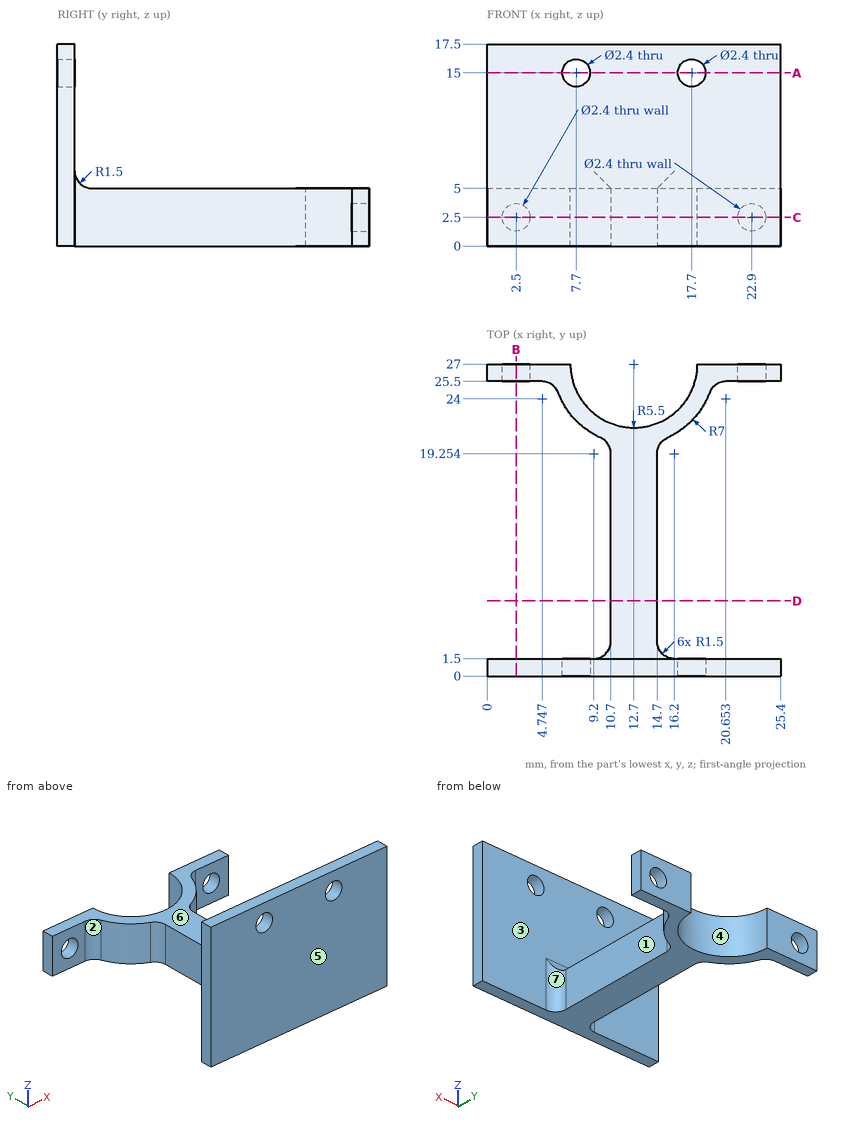
Geometry: see drawing. Coordinates: mm, zero at the bounding-box minimum. A direction names the side the tool comes from. Coordinates: 2 decimals unless noted, no trailing zeros. Order: outer loops, then holes, each group sorted by start corner. A loop starts at its lowest first (then second) coordinate and runs counter-clockwise, first axis right, second up. Notation, with made-up numbers: M 19,30.25 L 52,30.25 A10 cw 52,44.25 Z; hole C 3.5,79.5 d4. An arc over 180 degrees is marked long. Answer in a Markdown table with one row per item. Add a question column.
Q1. Section query D-D on y = 6.5. Return the cut outline in (x, z), and give its area (3 significant figures).
Q2. Section query B-B on x = 2.5. Return the cut outline in (y, z).
Q3. Contact query for flat-ended pins moving along their axis: P1, Ø5, axis at x = 4.5, z = 10, coming from the -Y side; P2, Ø1.5, axis at y = 12, z = 1.5, coming from the +X side; P3, Ø2, axis at x = 8.5, z = 11.5, coming from the +Y side; P4, Ø1.9, axis at x = 7.7, z = 15, coming from the +Y side. Output: stop coordinate, or through.
Q4. Mould query, pull axis Y, two halves, no side actions, for the marked faces 4, 5, 6 and 7. Classes: released by +Y, released by -Y, zero draft, split by the parting line, or undercut.
Q5. Line query: L1, parallel to X at y = 26.75, z = 2.5; L2, parallel to X at y = 0.4, z = 15; L3, parallel to Z at x = 2.5, y = 26.25. Output: solid intervals per line, ascending.
Q6. Section query A-A on z = 15. Return the cut outline in (x, y), and give its area (3 significant figures).
Q7. Section query C-C on z = 2.5. Count the separate pieces of the cut face and the enclosed holes in it, and give its area (3 significant figures).
Q8. Reachability of the marked faces 1, 2 and 3 from +Z, -Z, +X, -X, +Y, -Y: full face, straight path, thin tool, end or side. Return the list, or none.
Completed:
| question | item | result |
|---|---|---|
| 1 | outline | M 10.7,0 L 14.7,0 L 14.7,5 L 10.7,5 Z |
| 1 | area | 20.0 mm2 |
| 2 | outline | M 0,0 L 1.5,0 L 1.5,17.5 L 0,17.5 Z; M 25.5,0 L 27,0 L 27,1.3 L 25.5,1.3 Z; M 25.5,3.7 L 27,3.7 L 27,5 L 25.5,5 Z |
| 3 | P1 | stops at y = 0 |
| 3 | P2 | stops at x = 14.7 |
| 3 | P3 | stops at y = 1.5 |
| 3 | P4 | passes through |
| 4 | face 4 | released by +Y |
| 4 | face 5 | released by -Y |
| 4 | face 6 | zero draft |
| 4 | face 7 | undercut |
| 5 | L1 | x = 0 to 1.3, 3.7 to 7.21, 18.19 to 21.7, 24.1 to 25.4 |
| 5 | L2 | x = 0 to 6.5, 8.9 to 16.5, 18.9 to 25.4 |
| 5 | L3 | z = 0 to 1.3, 3.7 to 5 |
| 6 | outline | M 0,0 L 6.5,0 L 6.5,1.5 L 0,1.5 Z; M 8.9,0 L 16.5,0 L 16.5,1.5 L 8.9,1.5 Z; M 18.9,0 L 25.4,0 L 25.4,1.5 L 18.9,1.5 Z |
| 6 | area | 30.9 mm2 |
| 7 | separate pieces | 3 |
| 7 | enclosed holes | 0 |
| 7 | area | 154 mm2 |
| 8 | face 1 | +Z, -Z, +X |
| 8 | face 2 | +Z, -Z, -X |
| 8 | face 3 | +Z |
